Autodesk Inventor part; units mm, degrees
ref_plane "YZ Plane" through (0, 0, 0) normal (1, 0, 0) x (0, 1, 0)
ref_plane "XZ Plane" through (0, 0, 0) normal (0, 1, 0) x (-1, 0, 0)
ref_plane "XY Plane" through (0, 0, 0) normal (0, 0, 1) x (1, 0, 0)
sketch "Sketch1" plane through (0, 0, 0) normal (0, 0, 1) x (1, 0, 0)
  line L0 (-277.5467, 56.2236) -> (135.2033, 56.2236)
  line L1 (-277.5467, 56.2236) -> (-277.5467, 48.2861)
  line L2 (-277.5467, 48.2861) -> (-258.4967, 48.2861)
  line L3 (-258.4967, 48.2861) -> (-258.4967, 38.7611)
  line L4 (-258.4967, 38.7611) -> (-277.5467, 38.7611)
  line L5 (-277.5467, 38.7611) -> (-277.5467, 30.8236)
  line L6 (-277.5467, 30.8236) -> (135.2033, 30.8236)
  line L7 (135.2033, 30.8236) -> (135.2033, 38.7611)
  line L8 (135.2033, 38.7611) -> (116.1533, 38.7611)
  line L9 (116.1533, 38.7611) -> (116.1533, 48.2861)
  line L10 (116.1533, 48.2861) -> (135.2033, 48.2861)
  line L11 (135.2033, 48.2861) -> (135.2033, 56.2236)
  point P0 (0, 0)
  dimension "d0" = 412.75
  dimension "d1" = 7.9375
  dimension "d2" = 7.9375
  dimension "d3" = 9.525
  dimension "d4" = 7.9375
  dimension "d5" = 9.525
  dimension "d6" = 19.05
  dimension "d7" = 19.05
  dimension "d8" = 19.05
  dimension "d14" = 412.75
extrude "Extrusion1" add sketch "Sketch1" along normal blind 19.05
sketch "Sketch2" plane through (0, 0, 19.05) normal (0, 0, 1) x (1, 0, 0)
  line L0 (-258.4967, 48.2861) -> (116.1533, 48.2861)
  line L1 (116.1533, 48.2861) -> (116.1533, 38.7611)
  line L2 (116.1533, 38.7611) -> (-258.4967, 38.7611)
  line L3 (-258.4967, 38.7611) -> (-258.4967, 48.2861)
  point P0 (0, 0)
extrude "Extrusion2" cut sketch "Sketch2" against normal blind 9.525
equation "\"d14\" = d0"
properties part number "top_cover_end"
Input: part model. Units: mm. Frame: model coordinates. A direction names the side the tool comes from. Round coordinates to 2 decimals unless told otherwise and drop trailing zeros. Loops run counter-clockwise (first coordinate to the right, second up) from the corner with the lowest first, then second, coordinate; pieces in that order, holes last. Notation, with made-up numbers: (19.5, 19) -> (77.5, 19) arc R23 ccw to (77.5, 30) -> close; hole circle Ø9 at (11.25, -40). An arc over 180 degrees is marked (long way). One line per item, written item: value.
(1) Set-up query: faces 1 (the face through (-74, 56.224, 9)), 2 (the face through (-258.497, 44, 5)), 3 (the face through (116.153, 43, 5)), 4 (the face through (-74, 44, 9.525)). Return all of +Z, -Z, +X, -X, +Y, -Y with unobstructed straight access to the full face (end or side cutting, diameter ignored); none if empty.
Geometry check:
face 1: +Z, -Z, +X, -X, +Y
face 2: +Z, -Z, -X
face 3: +Z, -Z, +X
face 4: +Z, +X, -X
(2) Material intervals for line 1 (Y direction, x = 9, z = 11.25); line 2 (Z direction, x = -223, y = 43) (3 decimals); line 3 (X direction, y = 43.75, z = 7.75), sorted ascending. Write a range as [from, to].
Geometry check:
line 1: [30.82, 38.76], [48.29, 56.22]
line 2: [0, 9.525]
line 3: [-258.5, 116.15]
(3) Pin query (flat end, axial travel): pin 1 (5 mm diameter, centred on y = 42.5, z = 7, fed in from +X); pin 2 (7.5 mm diameter, centred on y = 43, z = 3, fed in from -X); pin 3 (1.5 mm diameter, centred on x = -141, y = 44, fed in from +Z) (3 decimals). Return the tip coordinate at first contact, or that it passes through.
Geometry check:
pin 1: x = 116.15
pin 2: x = -258.5
pin 3: z = 9.525
(4) Section B-B (x = 83). Return the cut outline in (y, z) (3 decimals).
Geometry check:
outline: (30.824, 0) -> (56.224, 0) -> (56.224, 19.05) -> (48.286, 19.05) -> (48.286, 9.525) -> (38.761, 9.525) -> (38.761, 19.05) -> (30.824, 19.05) -> close
(5) Section A-A (z = 13.5). Return the cut outline in (x, y).
Geometry check:
outline: (-277.55, 30.82) -> (135.2, 30.82) -> (135.2, 38.76) -> (-277.55, 38.76) -> close; (-277.55, 48.29) -> (135.2, 48.29) -> (135.2, 56.22) -> (-277.55, 56.22) -> close
(6) Mould query, pull axis Y, two halves, no side actions, for faces 5 (the face through (-74, 30.824, 9)), 6 (the face through (135.203, 35, 9)), 7 (the face through (-68, 38.761, 14)). Classes: pulls with the +Y half, pulls with the -Y half, needs draft (parallel to the pull), parting line crosses it, or undercut.
Geometry check:
face 5: pulls with the -Y half
face 6: needs draft
face 7: undercut
